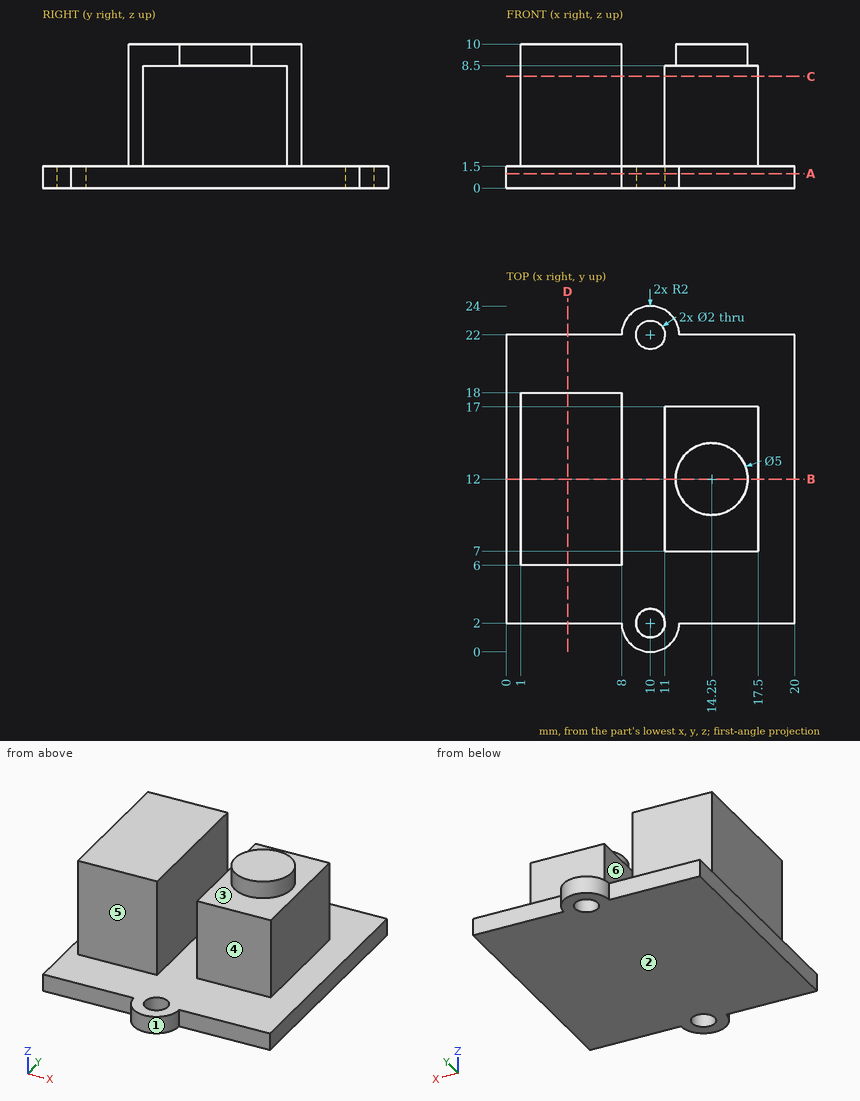
Geometry check sheet. Reference: drawing and pictorial views, mm from the part's lowest x, y, z. A direction names the side the tool comes from. Give positions to 0.01 mm unless a question says otherwise; leave off trailing zeros. Write each loop counter-clockwise with the first axis right and the second up, starting at its lowest first coordinate (ties: lowest second). Pieces come first, ordered by that corner, then holes. Notation, with made-up numbers: (57.25, -19.5) - (107.25, -19.5) arc R18 ccw to (107.25, 8.5) - close; hole circle Ø4 at (72, 55). An arc over 180 degrees is marked (long way). Use a Markdown table: item, result.
Q1. Draft check along X on the marked faces 1, 2 and 3. Enter one of: pulls with the +X half, pulls with the -X half, needs draft (parallel to the pull), parting line crosses it, or undercut.
Computed:
| item | result |
|---|---|
| face 1 | parting line crosses it |
| face 2 | needs draft |
| face 3 | undercut |
Q2. Go/stop test with flat-tipped pins: P1, Ø1, axis at y = 9, z = 5, coming from the +X side; P2, Ø5, axis at y = 13.5, z = 5.5, coming from the -X side; P3, Ø1.5, axis at x = 7.5, z = 6.5, coming from the -Y side; P4, Ø1.8, axis at x = 10, y = 22, coming from the -Z side. Record where each tip stops, or that it passes through.
Computed:
| item | result |
|---|---|
| P1 | stops at x = 17.5 |
| P2 | stops at x = 1 |
| P3 | stops at y = 6 |
| P4 | passes through |
Q3. Section check A-A, the plane z = 1. Enter the section's corners in (x, y).
Computed:
| item | result |
|---|---|
| outline | (0, 2) - (8, 2) arc R2 ccw to (12, 2) - (20, 2) - (20, 22) - (12, 22) arc R2 ccw to (8, 22) - (0, 22) - close; hole circle Ø2 at (10, 2); hole circle Ø2 at (10, 22) |
Q4. Set-up check for the marked faces 4, 5 and 6: record each of +Z, -Z, +X, -X, +Y, -Y from which the full face is reachable in a straight line by a thin tool's end or side.
Computed:
| item | result |
|---|---|
| face 4 | +Z, +X, -Y |
| face 5 | +Z, +X, -X, -Y |
| face 6 | +Z, +Y, -Y |
Q5. Section check C-C, the plane z = 7.75. Enter the section's corners in (x, y), then the cut area to 3 significant figures.
Computed:
| item | result |
|---|---|
| outline | (1, 6) - (8, 6) - (8, 18) - (1, 18) - close; (11, 7) - (17.5, 7) - (17.5, 17) - (11, 17) - close |
| area | 149 mm² |
Q6. Section check D-D, the plane x = 4.25. Enter the section's corners in (y, z).
Computed:
| item | result |
|---|---|
| outline | (2, 0) - (22, 0) - (22, 1.5) - (18, 1.5) - (18, 10) - (6, 10) - (6, 1.5) - (2, 1.5) - close |
Q7. Section check B-B, the plane y = 12. Enter the section's corners in (x, z).
Computed:
| item | result |
|---|---|
| outline | (0, 0) - (20, 0) - (20, 1.5) - (17.5, 1.5) - (17.5, 8.5) - (16.75, 8.5) - (16.75, 10) - (11.75, 10) - (11.75, 8.5) - (11, 8.5) - (11, 1.5) - (8, 1.5) - (8, 10) - (1, 10) - (1, 1.5) - (0, 1.5) - close |
Q8. Thickness scan on L1, parallel to Y at x = 10, z = 1; L2, parallel to X at y = 13.5, z = 3.5; L3, parallel to Z at x = 10.5, y = 11.25. Record the ranges inside material, lowest first. Write a range as [from, to].
Computed:
| item | result |
|---|---|
| L1 | y = [0, 1], [3, 21], [23, 24] |
| L2 | x = [1, 8], [11, 17.5] |
| L3 | z = [0, 1.5] |
